```python
from build123d import *

# Parameters (mm, degrees)
F0_R     = 11
F1_DEPTH = 7
F2_SIZE  = 1.5


with BuildPart() as f1:
    # F0 (on Top) → F1 (new body)
    with BuildSketch(Plane.XY):
        with BuildLine():
            ThreePointArc((10.2709292347, 9.5135699218), (11.240900909, 8.3451870413), (12.0786220303, 7.0786220303))
            Line((12.0786220303, 7.0786220303), (20, 15))
            Line((20, 15), (12.0786220303, 22.9213779697))
            ThreePointArc((12.0786220303, 22.9213779697), (11.240900909, 21.6548129587), (10.2709292347, 20.4864300782))
            Line((10.2709292347, 20.4864300782), (15.7573593129, 15))
            Line((15.7573593129, 15), (10.2709292347, 9.5135699218))
        make_face()
        with BuildLine():
            ThreePointArc((10.2709292347, 20.4864300782), (11.240900909, 21.6548129587), (12.0786220303, 22.9213779697))
            ThreePointArc((12.0786220303, 22.9213779697), (13.5111196506, 26.3326241278), (14, 30))
            ThreePointArc((14, 30), (-3.6673758722, 43.5111196506), (-12.0786220303, 22.9213779697))
            ThreePointArc((-12.0786220303, 22.9213779697), (-11.240900909, 21.6548129587), (-10.2709292347, 20.4864300782))
            ThreePointArc((-10.2709292347, 20.4864300782), (0, 16), (10.2709292347, 20.4864300782))
        make_face()
        with Locations((0, 30)):
            Circle(F0_R, mode=Mode.SUBTRACT)
        with BuildLine():
            ThreePointArc((-12.0786220303, 7.0786220303), (-11.240900909, 8.3451870413), (-10.2709292347, 9.5135699218))
            Line((-10.2709292347, 9.5135699218), (-15.7573593129, 15))
            Line((-15.7573593129, 15), (-10.2709292347, 20.4864300782))
            ThreePointArc((-10.2709292347, 20.4864300782), (-11.240900909, 21.6548129587), (-12.0786220303, 22.9213779697))
            Line((-12.0786220303, 22.9213779697), (-20, 15))
            Line((-20, 15), (-12.0786220303, 7.0786220303))
        make_face()
        with BuildLine():
            Line((-20.8690607132, 6.1462734615), (-13.3744578503, 4.1381006768))
            ThreePointArc((-13.3744578503, 4.1381006768), (-12.8475944316, 5.5623122279), (-12.1695775172, 6.9210825058))
            Line((-12.1695775172, 6.9210825058), (-22.9903810568, 9.8205080757))
            Line((-22.9903810568, 9.8205080757), (-25.8898066266, -1.0002954639))
            ThreePointArc((-25.8898066266, -1.0002954639), (-24.3740685909, -1.0925007307), (-22.8772334979, -1.3483294014))
            Line((-22.8772334979, -1.3483294014), (-20.8690607132, 6.1462734615))
        make_face()
        with BuildLine():
            ThreePointArc((3.1035286156, -13.6516705986), (10.9418782807, -8.7335731342), (14, 0))
            ThreePointArc((14, 0), (13.8427311233, 2.0925570597), (13.3744578503, 4.1381006768))
            ThreePointArc((13.3744578503, 4.1381006768), (12.8475944316, 5.5623122279), (12.1695775172, 6.9210825058))
            ThreePointArc((12.1695775172, 6.9210825058), (12.124355653, 7), (12.0786220303, 7.0786220303))
            ThreePointArc((12.0786220303, 7.0786220303), (11.240900909, 8.3451870413), (10.2709292347, 9.5135699218))
            ThreePointArc((10.2709292347, 9.5135699218), (0, 14), (-10.2709292347, 9.5135699218))
            ThreePointArc((-10.2709292347, 9.5135699218), (-11.240900909, 8.3451870413), (-12.0786220303, 7.0786220303))
            ThreePointArc((-12.0786220303, 7.0786220303), (-12.124355653, 7), (-12.1695775172, 6.9210825058))
            ThreePointArc((-12.1695775172, 6.9210825058), (-12.8475944316, 5.5623122279), (-13.3744578503, 4.1381006768))
            ThreePointArc((-13.3744578503, 4.1381006768), (-12.124355653, -7), (-3.1035286156, -13.6516705986))
            ThreePointArc((-3.1035286156, -13.6516705986), (-1.6066935226, -13.9074992693), (-0.0909554869, -13.9997045361))
            ThreePointArc((-0.0909554869, -13.9997045361), (0, -14), (0.0909554869, -13.9997045361))
            ThreePointArc((0.0909554869, -13.9997045361), (1.6066935226, -13.9074992693), (3.1035286156, -13.6516705986))
        make_face()
        Circle(F0_R, mode=Mode.SUBTRACT)
        with BuildLine():
            ThreePointArc((-25.8898066266, -1.0002954639), (-38.1051177665, -22), (-13.8111845963, -21.9210825058))
            ThreePointArc((-13.8111845963, -21.9210825058), (-13.1331676819, -20.5623122279), (-12.6063042633, -19.1381006768))
            ThreePointArc((-12.6063042633, -19.1381006768), (-12.1380309902, -17.0925570597), (-11.9807621135, -15))
            ThreePointArc((-11.9807621135, -15), (-15.0388838329, -6.2664268658), (-22.8772334979, -1.3483294014))
            ThreePointArc((-22.8772334979, -1.3483294014), (-24.3740685909, -1.0925007307), (-25.8898066266, -1.0002954639))
        make_face()
        with Locations((-25.9807621135, -15)):
            Circle(F0_R, mode=Mode.SUBTRACT)
        with BuildLine():
            Line((-2.9903810568, -24.8205080757), (-0.0909554869, -13.9997045361))
            ThreePointArc((-0.0909554869, -13.9997045361), (-1.6066935226, -13.9074992693), (-3.1035286156, -13.6516705986))
            Line((-3.1035286156, -13.6516705986), (-5.1117014003, -21.1462734615))
            Line((-5.1117014003, -21.1462734615), (-12.6063042633, -19.1381006768))
            ThreePointArc((-12.6063042633, -19.1381006768), (-13.1331676819, -20.5623122279), (-13.8111845963, -21.9210825058))
            Line((-13.8111845963, -21.9210825058), (-2.9903810568, -24.8205080757))
        make_face()
        with BuildLine():
            Line((5.1117014003, -21.1462734615), (3.1035286156, -13.6516705986))
            ThreePointArc((3.1035286156, -13.6516705986), (1.6066935226, -13.9074992693), (0.0909554869, -13.9997045361))
            Line((0.0909554869, -13.9997045361), (2.9903810568, -24.8205080757))
            Line((2.9903810568, -24.8205080757), (13.8111845963, -21.9210825058))
            ThreePointArc((13.8111845963, -21.9210825058), (13.1331676819, -20.5623122279), (12.6063042633, -19.1381006768))
            Line((12.6063042633, -19.1381006768), (5.1117014003, -21.1462734615))
        make_face()
        with BuildLine():
            ThreePointArc((12.1695775172, 6.9210825058), (12.8475944316, 5.5623122279), (13.3744578503, 4.1381006768))
            Line((13.3744578503, 4.1381006768), (20.8690607132, 6.1462734615))
            Line((20.8690607132, 6.1462734615), (22.8772334979, -1.3483294014))
            ThreePointArc((22.8772334979, -1.3483294014), (24.3740685909, -1.0925007307), (25.8898066266, -1.0002954639))
            Line((25.8898066266, -1.0002954639), (22.9903810568, 9.8205080757))
            Line((22.9903810568, 9.8205080757), (12.1695775172, 6.9210825058))
        make_face()
        with BuildLine():
            ThreePointArc((25.8898066266, -1.0002954639), (24.3740685909, -1.0925007307), (22.8772334979, -1.3483294014))
            ThreePointArc((22.8772334979, -1.3483294014), (13.8564064606, -8), (12.6063042633, -19.1381006768))
            ThreePointArc((12.6063042633, -19.1381006768), (13.1331676819, -20.5623122279), (13.8111845963, -21.9210825058))
            ThreePointArc((13.8111845963, -21.9210825058), (29.5602812683, -28.5346607871), (39.9807621135, -15))
            ThreePointArc((39.9807621135, -15), (35.8480470284, -5.0683995042), (25.8898066266, -1.0002954639))
        make_face()
        with Locations((25.9807621135, -15)):
            Circle(F0_R, mode=Mode.SUBTRACT)
    extrude(amount=F1_DEPTH)

    # F2
    f2_edges = [f1.edges().sort_by_distance(p)[0] for p in [
        (0, 44, 7),
        (-16.039311, 18.960689, 7),
        (-16.039311, 11.039311, 7),
        (-17.579979, 8.370795, 7),
        (-24.440094, 4.410106, 7),
        (-38.105118, -22, 7),
        (-8.400783, -23.370795, 7),
        (-1.540668, -19.410106, 7),
        (1.540668, -19.410106, 7),
        (8.400783, -23.370795, 7),
        (38.105118, -22, 7),
        (24.440094, 4.410106, 7),
        (17.579979, 8.370795, 7),
        (16.039311, 11.039311, 7),
        (16.039311, 18.960689, 7),
        (8.400783, -23.370795, 0),
        (24.440094, 4.410106, 0),
        (17.579979, 8.370795, 0),
        (16.039311, 11.039311, 0),
        (16.039311, 18.960689, 0),
        (0, 44, 0),
        (-16.039311, 18.960689, 0),
        (-16.039311, 11.039311, 0),
        (-17.579979, 8.370795, 0),
        (-24.440094, 4.410106, 0),
        (-38.105118, -22, 0),
        (-8.400783, -23.370795, 0),
        (-1.540668, -19.410106, 0),
        (1.540668, -19.410106, 0),
    ]]
    chamfer(f2_edges, length=F2_SIZE)


solid = f1.part
```
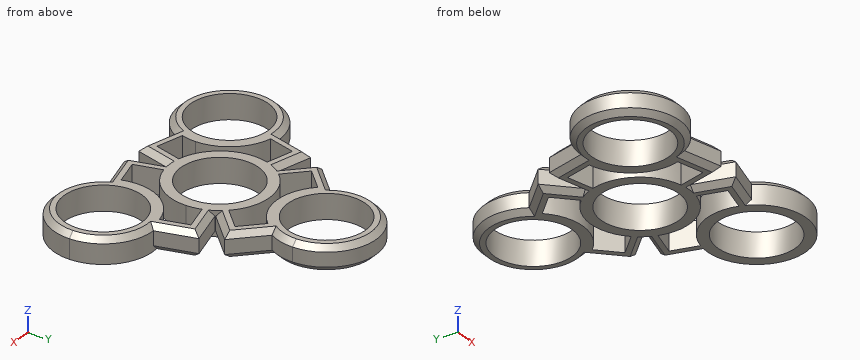
The listing builds one solid part. Answer for the finished solid, in the listing's coordinates (mm). Give positions to 0.01 mm unless a question says otherwise; leave off trailing zeros. Answer as a JSON object with one key per item and string values. Group by question number.
Item 1: Consider L1, parallel to Y at x = 0, z = 4.25; L2, parallel to X at y = -3, z = 3.5; L3, parallel to Y at x = -7, z = 6. Determine where each line is inside the solid, lowest interval first. Write a range as from..to.
Item 2: Flat-ended cylindrical pins translate along their axes: pin 1 (3 mm diameter, centred on y = -20, z = 2.5, fed in from -X); pin 2 (4 mm diameter, centred on y = -1, z = 4, fed in from +X); pin 3 (17.5 mm diameter, centred on x = 25.98, y = -15, fed in from -Z); pin 4 (4 mm diameter, centred on y = 33, z = 1, fed in from +X). Find the tip coordinate at first contact, or state that the pin passes through.
Item 3: The part is cut by section A-A on z = 3.5. Give the number of separate pieces and of enclosed holes in the cut face, and give its area (3 significant figures).
Result set:
{
 "1": {"L1": "-14..-11, 11..14, 16..19, 41..44", "L2": "-33.19..-18.77, -13.67..-10.58, 10.58..13.67, 18.77..33.19", "L3": "-23.23..-20.64, -12.12..-8.49, 8.49..12.12, 17.88..21.51, 38.49..41.54"},
 "2": {"pin 1": "x = -39.54", "pin 2": "x = 33.19", "pin 3": "through", "pin 4": "x = 13.96"},
 "3": {"separate pieces": "1", "enclosed holes": "7", "area": "1,280 mm²"}
}
